For this review, take the finished solid that the model builds, in its own axes (mm). A direction names the side the tool comes from. Coordinates: 2 decimals unless noted, no trailing zeros. Write each loop counter-clockwise with the first axis right and the second up, starting at its lowest first coordinate (ties: lowest second). Pieces come first, ordered by that corner, then holes. Notation, with made-up numbers: M 62.25,-14 L 95.25,-14 A16 ccw 95.25,-9 Z; hole C -11,30 d3. An arc over 180 degrees is marked long. Return JSON: item names as keys, results as strings.
```python
from build123d import *

# Parameters (mm, degrees)
F0_W     = 12.7
F0_H     = 12.7
F1_DEPTH = 25.4


with BuildPart() as f1:
    # F0 (on Front) → F1 (new body)
    with BuildSketch(Plane.XZ):
        with BuildLine():
            Line((-19.05, 88.9), (-19.05, 38.1))
            ThreePointArc((-19.05, 38.1), (-59.461153, 21.361153), (-76.2, -19.05))
            ThreePointArc((-76.2, -19.05), (-55.741409, -68.441409), (-6.35, -88.9))
            ThreePointArc((-6.35, -88.9), (52.021665, -64.721665), (76.2, -6.35))
            ThreePointArc((76.2, -6.35), (48.301921, 61.001921), (-19.05, 88.9))
        make_face()
        with Locations((-12.7, -12.7)):
            Rectangle(F0_W, F0_H, mode=Mode.SUBTRACT)
        with Locations((-12.7, -12.7)):
            Rectangle(F0_W, F0_H)
    extrude(amount=F1_DEPTH)


solid = f1.part
```
1. We need section B-B (z = -33). State the section outline as (x, y) points, plus the area to 3 significant figures.
Checks:
{"outline": "M -74.79,-25.4 L 71.78,-25.4 L 71.78,0 L -74.79,0 Z", "area": "3,720 mm2"}
2. We need section C-C (x = 63). State the section outline as (y, z) points, plus the area to 3 significant figures.
Checks:
{"outline": "M -25.4,-51.13 L 0,-51.13 L 0,42.03 L -25.4,42.03 Z", "area": "2,370 mm2"}
3. We need section A-A (y = -5). State the section outline as (x, z) points, plus the area to 3 significant figures.
Checks:
{"outline": "M -76.2,-19.05 A69.85 ccw -6.35,-88.9 A82.55 ccw 76.2,-6.35 A95.25 ccw -19.05,88.9 L -19.05,38.1 A57.15 ccw Z", "area": "19,000 mm2"}
4. Clearance check with flat-ended pins moving along their axes: pin 1 Ø2 at (y, z) = (-7, -45.5) entering from -X; pin 2 Ø6 at (y, z) = (-14, 3.5) entering from +X; pin 3 Ø2 at (x, y) = (44.5, -18) entering from +Z. State where each tip first meets the part, or that it passes through.
Checks:
{"pin 1": "x = -71.4", "pin 2": "x = 75.95", "pin 3": "z = 65.48"}
5. For faces 1 (the face through (-19.05, -13, 64)), 2 (the face through (51.376, -12.522, -65.36)), list the 3-axis set-ups (+Z, -Z, +X, -X, +Y, -Y) from which the entire face can be reached by the end or side of a thin tool; tool diameter is ignored.
Checks:
{"face 1": "+Z, -X, +Y, -Y", "face 2": "-Z, +X, +Y, -Y"}
6. Wall thickness on L1, parallel to Z at x = 39.5, y = -2.75; L2, parallel to X at y = -1.75, z = 8.5; L3, parallel to Z at x = -41, y = -18.75: over which ranges is each line inside the solid? List them lowest first. Write a range as from..to.
Checks:
{"L1": "-75..68.78", "L2": "-69.12..75.04", "L3": "-79.7..33.72"}
